The drawing under review shows one solid part. Ordinate dimensions are in mm from its lowest x, y, z. A direction names the side the tool comes from. Coordinates: 2 decimals unless noted, no trailing zeros. Order: outer loops, then holes, each group sorted by start corner. A loop starts at its lowest first (then second) coordinate and runs counter-clockwise, first axis right, second up.
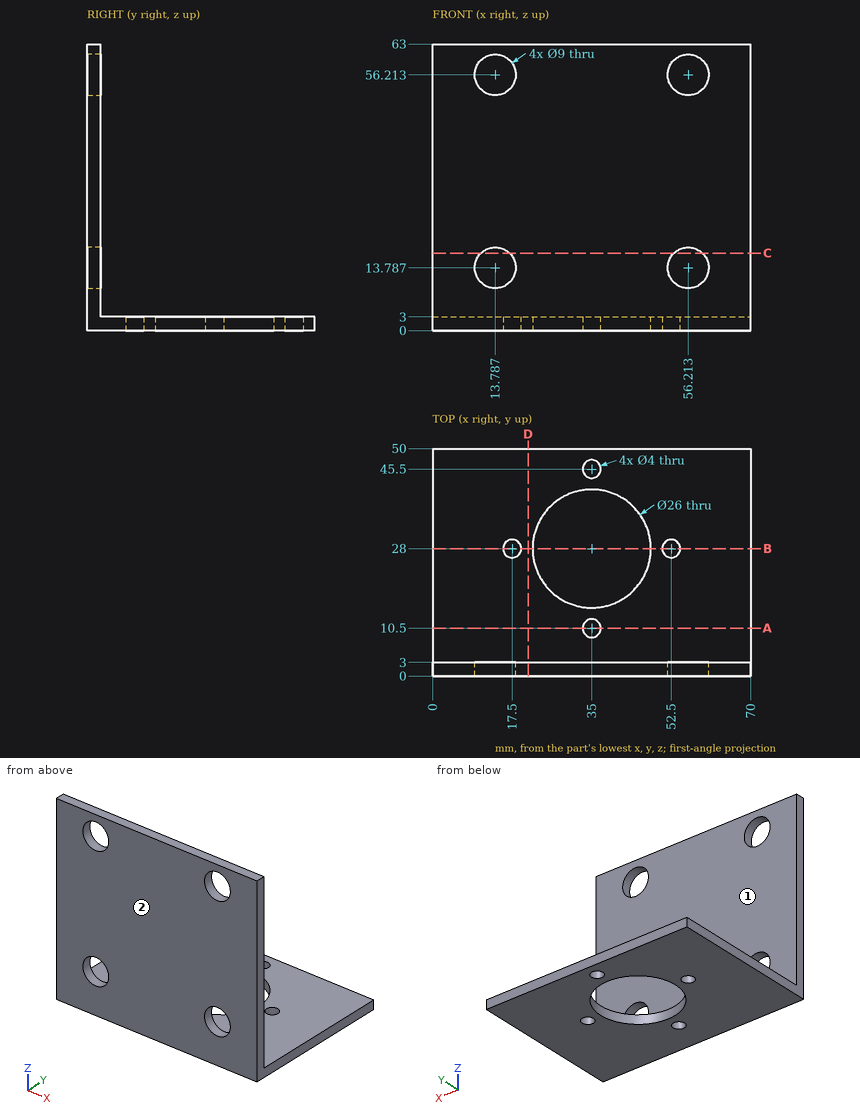
(1) Wall thickness on line 1 (Y direction, x = 35, z = 1.4); line 2 (Y direction, x = 17.5, z = 1.3); line 3 (Y direction, x = 45.5, z = 39): over which ranges is each line inside the solid? List them lowest first.
(2) Consider section A-A (y = 10.5). Give the boundary of the cut face in (x, z).
(3) Insertion check: pin 1 Ø5 at (x, y) = (17.5, 28) entering from +Z; pin 2 Ø1.5 at (x, z) = (55.5, 6.5) entering from +Y. Each pin has a flat end and moves straight along its axis. Give the tip position at first contact, or say it passes through.
(4) Consider section B-B (y = 28). Give the boundary of the cut face in (x, z), then the cut area to 3 significant figures.
(5) Consider section D-D (x = 21). Give the boundary of the cut face in (y, z).
(6) Tool access review of the marked faces 1 and 2: name each direction out of +Z, -Z, +X, -X, +Y, -Y from which nothing blocks a thin tool from reaching the whole face with its end or side.
(7) Consider section C-C (z = 17). Give the boundary of the cut face in (x, y).
Findings:
1. line 1: y = 0 to 8.5, 12.5 to 15, 41 to 43.5, 47.5 to 50
1. line 2: y = 0 to 26, 30 to 50
1. line 3: y = 0 to 3
2. outline: (0, 0) - (33, 0) - (33, 3) - (0, 3) - close; (37, 0) - (70, 0) - (70, 3) - (37, 3) - close
3. pin 1: stops at z = 3
3. pin 2: stops at y = 3
4. outline: (0, 0) - (15.5, 0) - (15.5, 3) - (0, 3) - close; (19.5, 0) - (22, 0) - (22, 3) - (19.5, 3) - close; (48, 0) - (50.5, 0) - (50.5, 3) - (48, 3) - close; (54.5, 0) - (70, 0) - (70, 3) - (54.5, 3) - close
4. area: 108 mm2
5. outline: (0, 0) - (50, 0) - (50, 3) - (3, 3) - (3, 63) - (0, 63) - close
6. face 1: +Z, +X, -X, +Y
6. face 2: +Z, -Z, +X, -X, -Y
7. outline: (0, 0) - (10.64, 0) - (10.64, 3) - (0, 3) - close; (16.94, 0) - (53.06, 0) - (53.06, 3) - (16.94, 3) - close; (59.36, 0) - (70, 0) - (70, 3) - (59.36, 3) - close
